Input: part model. Units: mm. Frame: model coordinates. Round coordinates to 2 decimals unless told otherwise and drop trailing zeros. Loops run counter-clockwise (first coordinate to the right, second up) from the corner with the lowest first, then second, coordinate; pieces in that order, holes last. Notation, with made-up numbers: (-37.75, 54.25) -> (-18.75, 54.25) arc R18 cw to (-18.75, 89.25) -> close; hole circle Ø9 at (16, 76). An arc over 180 degrees is marked (long way). Answer as a JSON object with one key per item and string values. Group by question number.
Item 1: Pin query (flat end, axial travel): pin 1 (13 mm diameter, centred on x = -12, z = 576.5, fed in from +Y); pin 2 (1 mm diameter, centred on x = 42.5, z = 366.5, fed in from +Y). Return the tip coordinate at first contact, or that it passes through.
Item 2: Section query B-B on x = -123.5. Return loops of the section in (y, z), and give its area (3 significant figures).
Item 3: Material intervals for line 1 (X direction, y = 582.5, z = 125.5); line 2 (Y direction, x = 143, z = 351.5), sorted ascending. Write a range as [from, to].
Item 4: Draft query along X for faces 1 (the flat face through (7, 18, 22)), 2 (the flat face through (500, -6, 296)), 3 (the flat face through (-420, 354, 301)), 4 (the flat face through (-400, 354, 301)). Return one class per face: released by +X, released by -X, zero draft, split by the parting line, or undercut.
Item 5: Section query A-A on z = 348.5. Return loops of the section in (x, y), and give its area (3 significant figures).
Item 6: Section query C-C on y = 265. Return loops of the section in (x, z), and give its area (3 significant figures).
from build123d import *

# Parameters (mm, degrees)
F0_W     = 1000
F0_H     = 600
F1_DEPTH = 15
F3_W     = 1000
F3_H     = 44
F4_DEPTH = 18
F5_W     = 1000
F5_H     = 44
F6_DEPTH = 18
F9_DEPTH = 20


with BuildPart() as f1:
    # F0 (on Front) → F1 (new body)
    with BuildSketch(Plane.XZ):
        with Locations((0, 300)):
            Rectangle(F0_W, F0_H)
    extrude(amount=F1_DEPTH)

    # F3 (on offset) → F4 (join)
    with BuildSketch(Plane(origin=(0, 0, 0), x_dir=(-1, 0, 0), z_dir=(0, 1, 0))):
        with Locations((0, 22)):
            Rectangle(F3_W, F3_H)
    extrude(amount=F4_DEPTH)

    # F5 (on offset) → F6 (join)
    with BuildSketch(Plane(origin=(0, 0, 0), x_dir=(-1, 0, 0), z_dir=(0, 1, 0))):
        with Locations((0, 578)):
            Rectangle(F5_W, F5_H)
    extrude(amount=F6_DEPTH)

    # F8 (on offset) → F9 (join)
    with BuildSketch(Plane(origin=(-400, 0, 0), x_dir=(0, -1, 0), z_dir=(-1, 0, 0))):
        Polygon((0, 503.4799401049), (0, 556), (-705, 96.5200598951), (-705, 44), align=None)
    extrude(amount=F9_DEPTH)

    # F10: F1 across plane


with BuildPart() as f1_1:
    add(f1.part)
    add(f1.part.mirror(Plane.YZ))


solid = f1_1.part
Solved:
{
 "1": {"pin 1": "y = 18", "pin 2": "y = 0"},
 "2": {"outline": "(-15, 0) -> (18, 0) -> (18, 44) -> (0, 44) -> (0, 556) -> (18, 556) -> (18, 600) -> (-15, 600) -> close", "area": "10,600 mm²"},
 "3": {"line 1": "[-420, -400], [400, 420]", "line 2": "[-15, 0]"},
 "4": {"face 1": "zero draft", "face 2": "released by +X", "face 3": "released by -X", "face 4": "undercut"},
 "5": {"outline": "(-500, -15) -> (500, -15) -> (500, 0) -> (-500, 0) -> close; (-420, 237.79) -> (-400, 237.79) -> (-400, 318.38) -> (-420, 318.38) -> close; (400, 237.79) -> (420, 237.79) -> (420, 318.38) -> (400, 318.38) -> close", "area": "18,200 mm²"},
 "6": {"outline": "(-420, 330.77) -> (-400, 330.77) -> (-400, 383.29) -> (-420, 383.29) -> close; (400, 330.77) -> (420, 330.77) -> (420, 383.29) -> (400, 383.29) -> close", "area": "2,100 mm²"}
}
